from build123d import *

# Parameters (mm, degrees)
SKETCH2_R           = 1.35
BOSS_EXTRUDE1_DEPTH = 3
SKETCH3_R           = 5
BOSS_EXTRUDE2_DEPTH = 3
SKETCH4_R           = 1.5
CUT_EXTRUDE1_DEPTH  = 4
SKETCH5_W           = 3
SKETCH5_H           = 20
SKETCH5_W_2         = 30
SKETCH5_H_2         = 3
BOSS_EXTRUDE3_DEPTH = 15


with BuildPart() as part:
    # Sketch2 → Boss-Extrude1 (new body)
    with BuildSketch(Plane(origin=(0, 0, 0), x_dir=(1, 0, 0), z_dir=(0, 1, 0))):
        Polygon((30, -55), (-30, -55), (-30, -30), (-55, -30), (-55, 30), (-30, 30), (-30, 55), (30, 55), (30, 30), (55, 30), (55, -30), (30, -30), align=None)
        with Locations((24.5, -42.5)):
            Circle(SKETCH2_R, mode=Mode.SUBTRACT)
        with Locations((-24.5, -42.5)):
            Circle(SKETCH2_R, mode=Mode.SUBTRACT)
        with Locations((24.5, 15.5)):
            Circle(SKETCH2_R, mode=Mode.SUBTRACT)
        with Locations((-24.5, 15.5)):
            Circle(SKETCH2_R, mode=Mode.SUBTRACT)
    extrude(amount=BOSS_EXTRUDE1_DEPTH)

    # Sketch3 → Boss-Extrude2 (add)
    with BuildSketch(Plane(origin=(0, 3, 0), x_dir=(1, 0, 0), z_dir=(0, 1, 0))):
        with Locations((50, 30)):
            Circle(SKETCH3_R)
        with Locations((50, -30)):
            Circle(SKETCH3_R)
        with Locations((-50, -30)):
            Circle(SKETCH3_R)
        with Locations((-50, 30)):
            Circle(SKETCH3_R)
    extrude(amount=-BOSS_EXTRUDE2_DEPTH)

    # Sketch4 → Cut-Extrude1 (cut, through all)
    with BuildSketch(Plane(origin=(0, 3, 0), x_dir=(1, 0, 0), z_dir=(0, 1, 0))):
        with Locations((50, 30)):
            Circle(SKETCH4_R)
        with Locations((50, -30)):
            Circle(SKETCH4_R)
        with Locations((-50, -30)):
            Circle(SKETCH4_R)
        with Locations((-50, 30)):
            Circle(SKETCH4_R)
    extrude(amount=-CUT_EXTRUDE1_DEPTH, mode=Mode.SUBTRACT)

    # Sketch5 → Boss-Extrude3 (add)
    with BuildSketch(Plane(origin=(0, 3, 0), x_dir=(1, 0, 0), z_dir=(0, 1, 0))):
        with Locations((-41.5, -8)):
            Rectangle(SKETCH5_W, SKETCH5_H)
        with Locations((41.5, -8)):
            Rectangle(SKETCH5_W, SKETCH5_H)
        with Locations((0, 11.5)):
            Rectangle(SKETCH5_W_2, SKETCH5_H_2)
        with Locations((0, -27.5)):
            Rectangle(SKETCH5_W_2, SKETCH5_H_2)
    extrude(amount=BOSS_EXTRUDE3_DEPTH)


solid = part.part
Can you work these out from the model? Positions are in its coordinate system, mm. A direction names the side the tool comes from. Give positions to 0.01 mm unless a question says otherwise; leave off trailing zeros. Order: outer loops, then holes, each group sorted by start corner. A loop starts at its lowest first (then second) coordinate and runs counter-clockwise, first axis right, second up. Notation, with made-up numbers: M -34.75,-17.75 L 10.25,-17.75 A7 ccw 10.25,-9.75 Z; hole C 34.25,32 d10. An arc over 180 degrees is marked long. Use one line per item in the form item = value. Start each with the question number.
Item 1: If we section it at C-C (z = -15.5): Write out the boundary of the cut face in (x, y), then the cut area to 3 significant figures.
Item 2: If we section it at D-D (y = 9.5): Write out the boundary of the cut face in (x, z).
Item 3: We'd pull the mould along Z, two halves only. Please class faces 5 (the flat face through (0, 10, -10)), 6 (the flat face through (41, 10, 18)), 7 (the flat face through (-42, 10, -2)): +Z half, -Z half, draft (parallel to the pull), parting line (faces both ways), or undercut.
Item 4: If I drill on line 1 along Z through (x, y) = (24.5, 0.65); line 2 along Z through (x, y) = (50, 0.9); line 3 along X through (y, z) = (1.45, -15.5), over which ranges is the centre line in solid material (lowest first)?
Item 5: If we section it at B-B (y = 1.5): State how many separate pieces and enclosed holes the cut face has, then the cut area to 3 significant figures.
Item 6: For faces 1 (the flat face through (0, 10, 26)), 2 (the flat face through (38, 1, 30)), 3 (the flat face through (40, 10, 8)), 4 (the flat face through (37, 1, -30)), which set-ups out of +Z, -Z, +X, -X, +Y, -Y let a thin tool reach every point of the face, with its end or its side?
Item 7: Will these pins go through, and if not, where does the flat tip stop? pin 1 Ø4 at (x, z) = (13.5, 8) entering from -Y; pin 2 Ø3.5 at (x, z) = (-50, 30) entering from +Y; pin 3 Ø1.5 at (x, y) = (41, 14) entering from +Z; pin 4 Ø0.9 at (y, z) = (2, -48) entering from +X.
Item 8: If we section it at A-A (x = 24.5): Write out the boundary of the cut face in (y, z), then the cut area to 3 significant figures.
Outcome:
q1.outline = M -55,0 L -25.85,0 L -25.85,3 L -55,3 Z; M -23.15,0 L 23.15,0 L 23.15,3 L -23.15,3 Z; M 25.85,0 L 55,0 L 55,3 L 25.85,3 Z
q1.area = 314 mm2
q2.outline = M -43,-2 L -40,-2 L -40,18 L -43,18 Z; M -15,-13 L 15,-13 L 15,-10 L -15,-10 Z; M -15,26 L 15,26 L 15,29 L -15,29 Z; M 40,-2 L 43,-2 L 43,18 L 40,18 Z
q3.face_5 = undercut
q3.face_6 = +Z half
q3.face_7 = -Z half
q4.line_1 = -55 to -16.85, -14.15 to 41.15, 43.85 to 55
q4.line_2 = -35 to -31.5, -28.5 to 28.5, 31.5 to 35
q4.line_3 = -55 to -25.85, -23.15 to 23.15, 25.85 to 55
q5.separate_pieces = 1
q5.enclosed_holes = 8
q5.area = 9,710 mm2
q6.face_1 = +X, -X, +Y
q6.face_2 = +Z, +Y, -Y
q6.face_3 = +Z, -Z, +Y
q6.face_4 = -Z, +Y, -Y
q7.pin_1 = 0
q7.pin_2 = 3
q7.pin_3 = 18
q7.pin_4 = 30
q8.outline = M 0,-55 L 3,-55 L 3,-16.85 L 0,-16.85 Z; M 0,-14.15 L 3,-14.15 L 3,41.15 L 0,41.15 Z; M 0,43.85 L 3,43.85 L 3,55 L 0,55 Z
q8.area = 314 mm2
